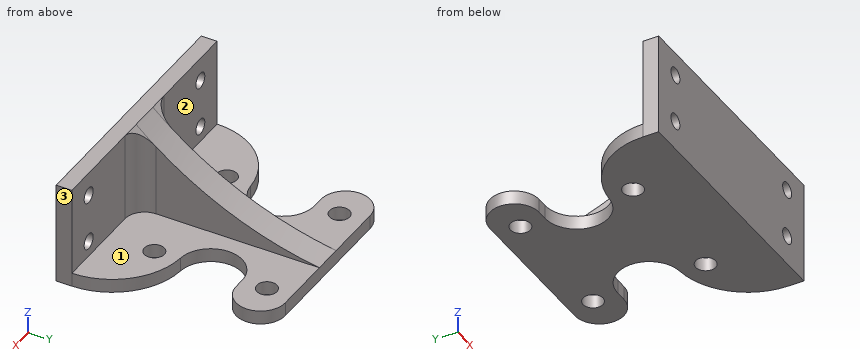
```python
from build123d import *

# Parameters (mm, degrees)
SKETCH1_W               = 130
SKETCH1_H               = 120
BOSS_EXTRUDE1_DEPTH     = 7
SKETCH2_R               = 13.462
SKETCH2_R_2             = 5.08
CUT_EXTRUDE1_DEPTH      = 89.735562206
SKETCH4_W               = 130
SKETCH4_H               = 8
BOSS_EXTRUDE2_DEPTH     = 45
CUT_EXTRUDE4_START      = -10
SKETCH10_R              = 13.462
CUT_EXTRUDE4_DEPTH      = 10
SKETCH11_R              = 4
CUT_EXTRUDE5_DEPTH      = 125.811858411
RIB1_REACH              = 104.611
SKETCH9_WALL_W          = 310.536883344
SKETCH9_WALL_H          = 15
CUT_EXTRUDE6_DEPTH      = 108.518603042
CUT_EXTRUDE6_DEPTH_BACK = 108.518603042
FILLET1_R               = 10


with BuildPart() as part:
    # Sketch1 → Boss-Extrude1 (new body)
    with BuildSketch(Plane.XY):
        Rectangle(SKETCH1_W, SKETCH1_H)
    extrude(amount=BOSS_EXTRUDE1_DEPTH)

    # Sketch2 → Cut-Extrude1 (cut, through all)
    with BuildSketch(Plane.XY.offset(7)):
        with Locations((-32.5, 0)):
            Circle(SKETCH2_R)
        with Locations((-32.5, 28.575)):
            Circle(SKETCH2_R_2)
        with Locations((-32.5, -28.575)):
            Circle(SKETCH2_R_2)
        with Locations(Location((32.5, -28.575, 0), (0, 0, 180))):
            Circle(SKETCH2_R_2)
        with Locations(Location((32.5, 0, 0), (0, 0, 180))):
            Circle(SKETCH2_R)
        with Locations(Location((32.5, 28.575, 0), (0, 0, 180))):
            Circle(SKETCH2_R_2)
    extrude(amount=-CUT_EXTRUDE1_DEPTH, mode=Mode.SUBTRACT)

    # Sketch4 → Boss-Extrude2 (add)
    with BuildSketch(Plane.XY.offset(7)):
        with Locations((0, -56)):
            Rectangle(SKETCH4_W, SKETCH4_H)
    extrude(amount=BOSS_EXTRUDE2_DEPTH)

    # Sketch10 → Cut-Extrude4 (cut)
    with BuildSketch(Plane(origin=(0, 0, 0), x_dir=(-1, 0, 0), z_dir=(0, 0, -1)).offset(CUT_EXTRUDE4_START)):
        with BuildLine():
            ThreePointArc((31.386922126, -15.961236094), (55.292470874, -27.359426204), (65, -52))
            Line((65, -52), (65, 60))
            Line((65, 60), (-65, 60))
            Line((-65, 60), (-65, -52))
            ThreePointArc((-65, -52), (-55.292470874, -27.359426204), (-31.386922126, -15.961236094))
            ThreePointArc((-31.386922126, -15.961236094), (-16.509693913, 0.556876331), (-32.5, 16))
            Line((-32.5, 16), (-38, 16))
            ThreePointArc((-38, 16), (-50.5, 28.5), (-38, 41))
            Line((-38, 41), (38, 41))
            ThreePointArc((38, 41), (50.5, 28.5), (38, 16))
            Line((38, 16), (32.5, 16))
            ThreePointArc((32.5, 16), (16.509693913, 0.556876331), (31.386922126, -15.961236094))
        make_face()
        with Locations((-32.5, 0)):
            Circle(SKETCH10_R, mode=Mode.SUBTRACT)
        with Locations((32.5, 0)):
            Circle(SKETCH10_R, mode=Mode.SUBTRACT)
    extrude(amount=CUT_EXTRUDE4_DEPTH, mode=Mode.SUBTRACT)

    # Sketch11 → Cut-Extrude5 (cut, through all)
    with BuildSketch(Plane(origin=(0, -52, 0), x_dir=(1, 0, 0), z_dir=(0, 1, 0))):
        with Locations(Location((-50, -15, 0), (0, 0, 180))):
            Circle(SKETCH11_R)
        with Locations(Location((-50, -40, 0), (0, 0, 180))):
            Circle(SKETCH11_R)
        with Locations((50, -40)):
            Circle(SKETCH11_R)
        with Locations((50, -15)):
            Circle(SKETCH11_R)
    extrude(amount=-CUT_EXTRUDE5_DEPTH, mode=Mode.SUBTRACT)

    # Sketch9 wall → Rib1 (add, up to next)
    with BuildSketch(Plane(origin=(0, -5.5, 29.5), x_dir=(0, -0.900159251416, 0.435560928104), z_dir=(0, -0.435560928104, -0.900159251416)), mode=Mode.PRIVATE) as rib1_sk1:
        Rectangle(SKETCH9_WALL_W, SKETCH9_WALL_H)
    rib1_tool1 = extrude(rib1_sk1.sketch, amount=RIB1_REACH, mode=Mode.PRIVATE) - part.part
    add(rib1_tool1.solids().sort_by_distance((0, -5.5, 29.5))[0])

    # Sketch13 → Cut-Extrude6 (cut, two sides: drawn at the far end of the back side and taken through both)
    with BuildSketch(Plane(origin=(7.5, 0, 0), x_dir=(0, 0, -1), z_dir=(1, 0, 0)).offset(-CUT_EXTRUDE6_DEPTH_BACK)):
        with BuildLine():
            ThreePointArc((-7, 41), (-22.684215539, -8.797960223), (-52, -52))
            Line((-52, -52), (-7, 41))
        make_face()
    extrude(amount=CUT_EXTRUDE6_DEPTH + CUT_EXTRUDE6_DEPTH_BACK, mode=Mode.SUBTRACT)

    # Fillet1
    # the kernel refuses this fillet: 10 mm, written as the material it adds along each edge
    with BuildSketch(Plane(origin=(7.5, -52, 7), x_dir=(1, 0, 0), z_dir=(0, 0, 1))) as fillet1_piece_1_section:
        with BuildLine():
            CenterArc((FILLET1_R, FILLET1_R), FILLET1_R, 180, 90)
            Line((0, FILLET1_R), (0, 0))
            Line((0, 0), (FILLET1_R, 0))
        make_face()
    fillet1_piece_1 = extrude(amount=45, mode=Mode.PRIVATE)
    fillet1_piece_1 = fillet1_piece_1 - Plane(origin=(9.819534596, 69.603006836, 184.712880794), x_dir=(0, -0.15890559353119482, -0.9872937821866897), z_dir=(-1, 0, 0)) * Cylinder(180, 130, mode=Mode.PRIVATE)
    add(fillet1_piece_1)
    with BuildSketch(Plane(origin=(-7.5, -52, 52), x_dir=(-1, 0, 0), z_dir=(0, 0, -1))) as fillet1_piece_2_section:
        with BuildLine():
            CenterArc((FILLET1_R, FILLET1_R), FILLET1_R, 180, 90)
            Line((0, FILLET1_R), (0, 0))
            Line((0, 0), (FILLET1_R, 0))
        make_face()
    fillet1_piece_2 = extrude(amount=45, mode=Mode.PRIVATE)
    fillet1_piece_2 = fillet1_piece_2 - Plane(origin=(-9.819536327, 69.603006836, 184.712880794), x_dir=(0, -0.15890559353119482, -0.9872937821866897), z_dir=(-1, 0, 0)) * Cylinder(180, 130, mode=Mode.PRIVATE)
    add(fillet1_piece_2)


solid = part.part
```
Verification items for the finished model (mm, model axes). Face numbers are marked on the shaded views. A direction names the side the tool comes from. Coordinates: 2 decimals unless noted, no trailing zeros. Loops run counter-clockwise (first coordinate to the right, second up) from the corner with the lowest first, then second, coordinate; pieces in that order, holes last. Notation, with made-up numbers: (87.25, 88) - (95.25, 88) arc R17 ccw to (95.25, 98) - close; hole circle Ø3 at (15, 34). An arc over 180 degrees is marked (long way). Return JSON: item names as keys, results as strings.
1. Section check C-C, the plane z = 4.5. Record the boundary of the cut face in (x, y) (3 decimals).
Established:
{"outline": "(-65, -60) - (65, -60) - (65, -52) arc R36.126 ccw to (31.387, -15.961) arc R16 cw to (32.5, 16) - (38, 16) arc R12.5 ccw to (38, 41) - (-38, 41) arc R12.5 ccw to (-38, 16) - (-32.5, 16) arc R16 cw to (-31.387, -15.961) arc R36.126 ccw to (-65, -52) - close; hole circle Ø10.16 at (-32.5, -28.575); hole circle Ø10.16 at (-32.5, 28.575); hole circle Ø10.16 at (32.5, -28.575); hole circle Ø10.16 at (32.5, 28.575)"}
2. Section check D-D, the plane y = -9. Record the boundary of the cut face in (x, z).
Established:
{"outline": "(-19.27, 0) - (19.27, 0) - (19.27, 7) - (7.5, 7) - (7.5, 22.78) - (-7.5, 22.78) - (-7.5, 7) - (-19.27, 7) - close"}
3. Go/stop test with flat-tipped pins: pin 1 (10 mm diameter, centred on y = -33.5, z = 21.5, fed in from +X); pin 2 (2 mm diameter, centred on y = -34.5, z = 10.5, fed in from -X); pin 3 (13 mm diameter, centred on x = 50, z = 15, fed in from +Y). Record where each tip stops, or that it passes through.
Established:
{"pin 1": "stops at x = 7.5", "pin 2": "stops at x = -7.5", "pin 3": "stops at y = -52"}
4. Tool access check on the marked faces 1, 2 and 3. Record the directions out of +Z, -Z, +X, -X, +Y, -Y that give a thin tool (end or side, any length) a straight path to the whole face; none if there is none.
Established:
{"face 1": "+Z, +X, +Y", "face 2": "+Z, -X, +Y", "face 3": "+Z, -Z, +X, +Y, -Y"}
5. Section check B-B, the plane x = 40. Record the boundary of the cut face in (y, z).
Established:
{"outline": "(-60, 0) - (-17.63, 0) - (-17.63, 7) - (-52, 7) - (-52, 52) - (-60, 52) - close; (16.16, 0) - (40.84, 0) - (40.84, 7) - (16.16, 7) - close"}
6. Section check A-A, the plane z = 15. Record the boundary of the cut face in (x, y), then the cut area to 3 significant figures.
Established:
{"outline": "(-65, -60) - (-54, -60) - (-54, -52) - (-65, -52) - close; (-46, -60) - (46, -60) - (46, -52) - (17.5, -52) arc R10 cw to (7.5, -42) - (7.5, 9.62) - (-7.5, 9.62) - (-7.5, -42) arc R10 cw to (-17.5, -52) - (-46, -52) - close; (54, -60) - (65, -60) - (65, -52) - (54, -52) - close", "area": "1,880 mm2"}
7. Thickness scan on L1, parallel to Z at x = -50, y = -55; L2, parallel to Y at x = -32.5, z = 3.75 (3 decimals); L3, parallel to Y at x = 45, z = 35.5. Record the ranges inside material, lowest first.
Established:
{"L1": "z = 0 to 11, 19 to 36, 44 to 52", "L2": "y = -60 to -33.655, -23.495 to -16.056, 16 to 23.495, 33.655 to 41", "L3": "y = -60 to -52"}
